For this review, take the finished solid that the model builds, in its own axes (mm). Face numbers are marked on the shaded views. A direction names the side the tool comes from. Round coordinates to 2 decimals unless told otherwise and drop trailing zeros. Write each loop counter-clockwise with the first axis right and the second up, starting at its lowest first coordinate (ties: lowest second). Pieces come first, ordered by that corner, then holes. Notation, with made-up numbers: M -22.5,50 L 0.5,50 A26 cw 0.5,74 Z; hole C 5.5,15.25 d10. An arc over 180 degrees is marked long. Answer in a Markdown table with one row per item.
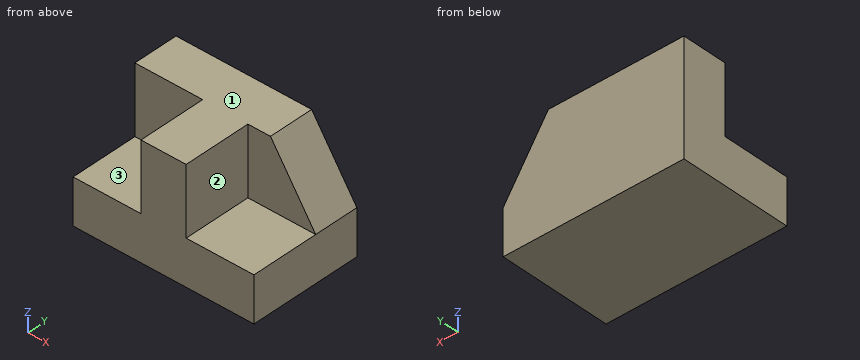
```python
from build123d import *

# Parameters (mm, degrees)
F0_W     = 50.8
F0_H     = 31.75
F1_DEPTH = 31.75
F2_W     = 19.05
F2_H     = 19.05
F3_DEPTH = 19.05
F4_W     = 19.05
F4_H     = 19.05
F5_DEPTH = 19.05
F7_DEPTH = 12.7


with BuildPart() as f1:
    # F0 (on Front) → F1 (new body)
    with BuildSketch(Plane.XZ):
        with Locations((-25.4, 15.875)):
            Rectangle(F0_W, F0_H)
    extrude(amount=F1_DEPTH)

    # F2 (on face) → F3 (cut)
    with BuildSketch(Plane.XY.offset(31.75)):
        with Locations((-9.525, -22.225)):
            Rectangle(F2_W, F2_H)
    extrude(amount=-F3_DEPTH, mode=Mode.SUBTRACT)

    # F4 (on face) → F5 (cut)
    with BuildSketch(Plane.XZ.offset(31.75)):
        with Locations((-41.275, 22.225)):
            Rectangle(F4_W, F4_H)
    extrude(amount=-F5_DEPTH, mode=Mode.SUBTRACT)

    # F6 (on face) → F7 (cut)
    with BuildSketch(Plane.XZ.offset(12.7)):
        Polygon((0, 31.75), (-12.7, 31.75), (0, 12.7), align=None)
    extrude(amount=-F7_DEPTH, mode=Mode.SUBTRACT)


solid = f1.part
```
Q1. Take a section at C-C (z = 23.5). State the section outline as (x, y) points.
Found:
| item | result |
|---|---|
| outline | M -50.8,-12.7 L -31.75,-12.7 L -31.75,-31.75 L -19.05,-31.75 L -19.05,-12.7 L -7.2,-12.7 L -7.2,0 L -50.8,0 Z |
Q2. Take a section at D-D (y = -19.5). State the section outline as (x, z) points, then the cut area to 3 significant figures.
Found:
| item | result |
|---|---|
| outline | M -50.8,0 L 0,0 L 0,12.7 L -19.05,12.7 L -19.05,31.75 L -31.75,31.75 L -31.75,12.7 L -50.8,12.7 Z |
| area | 887 mm² |
Q3. For probe 1 along X at (y, z) = (-25.5, 24.5); probe 2 along Z at (x, y) = (-14.5, -26); probe 3 along Y at (x, z) = (-16.5, 27), list the stretches that pass through material, from the lowest coordinate up.
Found:
| item | result |
|---|---|
| probe 1 | -31.75 to -19.05 |
| probe 2 | 0 to 12.7 |
| probe 3 | -12.7 to 0 |
Q4. Take a section at A-A (x = -34). State the section outline as (y, z) points, then the cut area to 3 significant figures.
Found:
| item | result |
|---|---|
| outline | M -31.75,0 L 0,0 L 0,31.75 L -12.7,31.75 L -12.7,12.7 L -31.75,12.7 Z |
| area | 645 mm² |
Q5. Insertion check: P1, Ø15, axis at x = -45.5, z = 21.5, coming from the -Y side; P2, Ø15, axis at y = -21, z = 21, coming from the -X side; P3, Ø2, axis at x = -11.5, y = -14, coming from the +Z side. Each pin has a flat end and moves straight along its axis. Give the tip position at first contact, or say it passes through.
Found:
| item | result |
|---|---|
| P1 | y = -12.7 |
| P2 | x = -31.75 |
| P3 | z = 12.7 |
Q6. Machinability: for the marked faces 1, 2 and 3, which of the approach directions +Z, -Z, +X, -X, +Y, -Y give a long, thin tool a straight path to every point of the face, cutting with its end or side? Answer none if there is none.
Found:
| item | result |
|---|---|
| face 1 | +Z, +X, -X, +Y, -Y |
| face 2 | +Z, +X, -Y |
| face 3 | +Z, -X, -Y |
Q7. Take a section at B-B (y = -9.5). State the section outline as (x, z) points, then the cut area to 3 significant figures.
Found:
| item | result |
|---|---|
| outline | M -50.8,0 L 0,0 L 0,12.7 L -12.7,31.75 L -50.8,31.75 Z |
| area | 1,490 mm² |
